Autodesk Inventor part; units mm, degrees
ref_plane "Work Plane1" through (-25.4, 0, 6.35) normal (0, 0, 1) x (1, 0, 0)
ref_plane "YZ Plane" through (0, 0, 0) normal (1, 0, 0) x (0, 1, 0)
ref_plane "XZ Plane" through (0, 0, 0) normal (0, 1, 0) x (-1, 0, 0)
sketch "Sketch1" plane through (0, 0, 0) normal (0, 1, 0) x (-1, 0, 0)
  line L0 (0, 0) -> (25.4, 0)
  line L1 (25.4, 0) -> (25.4, 12.7)
  line L2 (25.4, 12.7) -> (0, 12.7)
  line L3 (0, 12.7) -> (0, 0)
  line L4 (3.175, 9.525) -> (22.225, 9.525)
  line L5 (22.225, 9.525) -> (22.225, 3.175)
  line L6 (22.225, 3.175) -> (3.175, 3.175)
  line L7 (3.175, 3.175) -> (3.175, 9.525)
  dimension "d0" = 25.4
  dimension "d2" = 3.175
  dimension "d5" = 12.7
extrude "Extrusion1" add sketch "Sketch1" along normal blind 660.4
sketch "Sketch2" plane through (-25.4, 0, 12.7) normal (0, 0, 1) x (1, 0, 0)
  circle A0 centre (12.7, 41.275) radius 3.3782
  circle A1 centre (12.7, 22.225) radius 3.3782
  circle A2 centre (12.7, 619.125) radius 3.3782
  circle A3 centre (12.7, 638.175) radius 3.3782
  line L0 (25.4, 0) -> (0, 0)
  line L1 (25.4, 660.4) -> (25.4, 0)
  line L2 (0, 660.4) -> (25.4, 660.4)
  line L3 (0, 0) -> (0, 660.4)
extrude "Extrusion2" cut sketch "Sketch2" against normal blind 25.4 contours A0 | A1 | A2 | A3
ref_plane "Work Plane1" through (-25.4, 0, 6.35) normal (0, 0, 1) x (1, 0, 0)
sketch "Sketch3" plane through (0, 0, 0) normal (1, 0, 0) x (0, 0, -1)
  line L0 (-12.7, 0) -> (0, 0)
  line L1 (-12.7, 660.4) -> (0, 660.4)
  line L2 (-6.35, 0) -> (-6.35, 660.4) construction
  circle A0 centre (-6.35, 647.7) radius 3.175
  circle A1 centre (-6.35, 628.65) radius 3.175
  circle A2 centre (-6.35, 12.7) radius 3.175
  circle A3 centre (-6.35, 31.75) radius 3.175
  dimension "d8" = 6.35
  dimension "d10" = 12.7
  dimension "d11" = 19.05
  dimension "d12" = 12.7
  dimension "d13" = 19.05
extrude "Extrusion3" cut sketch "Sketch3" against normal blind 25.4
properties part number "M - 26 inch rail" material "Aluminum 6061"
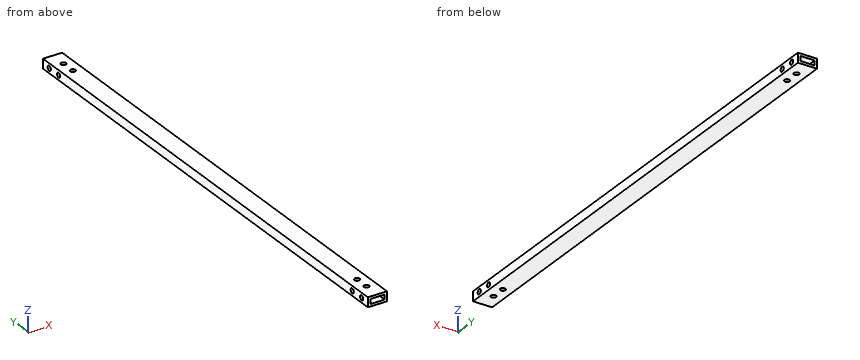
CAD build for the part. Positions are in the model's coordinates, mm. Coordinates: 2 decimals unless noted, no trailing zeros. Write each loop counter-clockwise with the first axis right and the second up, starting at its lowest first coordinate (ties: lowest second). Pieces come first, ordered by that corner, then holes. Notation, with made-up numbers: (67.25, 0) -> (123.25, 0) arc R17 cw to (123.25, 24) -> close; hole circle Ø6 at (-10, 52). An arc over 180 degrees is marked (long way). Return JSON: item names as keys, results as strings. Group by question number.
Q1. Drill centre lines: line 1 (Y direction, x = -23.55, z = 6.35) (3 decimals); line 2 (Z direction, x = -15.75, y = 479) (3 decimals); line 3 (Y direction, x = -12.7, z = 1.65). Where is each one in solid material? Low to high.
Q2. Flat gauge pin, fed straight in: pin 1 (5.5 mm diameter, centred on y = 647.7, z = 6.35, fed in from -X). Where does the tip first touch, or does it go through?
Q3. Cut at A-A, the plane y = 298. Give the cut face in (x, z) (3 decimals).
Q4. Cut at B-B, the plane z = 6.75. State how many separate pieces and enclosed holes the cut face has, then the cut area to 3 significant figures.
Returned:
{
 "1": {"line 1": "y = 0 to 9.525, 15.875 to 28.575, 34.925 to 625.475, 631.825 to 644.525, 650.875 to 660.4", "line 2": "z = 0 to 3.175, 9.525 to 12.7", "line 3": "y = 0 to 18.85, 25.6 to 37.9, 44.65 to 615.75, 622.5 to 634.8, 641.55 to 660.4"},
 "2": {"pin 1": "passes through"},
 "3": {"outline": "(-25.4, 0) -> (0, 0) -> (0, 12.7) -> (-25.4, 12.7) -> close; hole (-22.225, 3.175) -> (-3.175, 3.175) -> (-3.175, 9.525) -> (-22.225, 9.525) -> close"},
 "4": {"separate pieces": "10", "enclosed holes": "0", "area": "4,030 mm2"}
}
